Could you check a few things on this model? Use its own coordinates, in mm. A direction names the side the tool comes from. Give positions to 0.01 mm unless a question says otherwise; leave off trailing zeros. Order: outer loops, then holes, each group sorted by start corner. A loop starts at its lowest first (then second) coordinate and runs counter-clockwise, first axis right, second up. Notation, with made-up numbers: (37.5, 11.5) -> (85.5, 11.5) arc R19 ccw to (85.5, 39.5) -> close; hole circle Ø5 at (-23, -12). An arc over 180 degrees is marked (long way). Use one line per item in the form item = value. Start each with the question number.
from build123d import *

# Parameters (mm, degrees)
SKETCH1_R           = 76.2
BOSS_EXTRUDE1_DEPTH = 16.256
SHELL1_T            = -3.175
FILLET1_R           = 1.5875
SKETCH2_R           = 38.1
CUT_EXTRUDE1_DEPTH  = 16.256
SKETCH3_R           = 1.524
CUT_EXTRUDE2_DEPTH  = 76.2
CIRPATTERN1_COUNT   = 6
CUT_EXTRUDE4_START  = -1.524
SKETCH5_R           = 76.2
CUT_EXTRUDE4_DEPTH  = 1.524


with BuildPart() as part:
    # Sketch1 → Boss-Extrude1 (new body)
    with BuildSketch(Plane(origin=(0, 0, 0), x_dir=(1, 0, 0), z_dir=(0, 1, 0))):
        with Locations(Location((0, 0, 0), (0, 0, 270))):
            Circle(SKETCH1_R)
    extrude(amount=BOSS_EXTRUDE1_DEPTH)

    # Shell1
    shell1_openings = [part.faces().sort_by_distance(p)[0] for p in [
        (0, 16.256, 0),
    ]]
    offset(amount=SHELL1_T, openings=shell1_openings, kind=Kind.INTERSECTION)

    # Fillet1
    fillet1_edges = [part.edges().sort_by_distance(p)[0] for p in [
        (0, 3.175, -73.025),
    ]]
    fillet(fillet1_edges, radius=FILLET1_R)

    # Sketch2 → Cut-Extrude1 (cut)
    with BuildSketch(Plane.XZ):
        with Locations(Location((0, 0, 0), (0, 0, 270))):
            Circle(SKETCH2_R)
    extrude(amount=-CUT_EXTRUDE1_DEPTH, mode=Mode.SUBTRACT)

    # Sketch3 → Cut-Extrude2 (cut)
    with BuildSketch(Plane(origin=(0, 0, 0), x_dir=(0, 0, -1), z_dir=(1, 0, 0))):
        with Locations((0, 8.636)):
            Circle(SKETCH3_R)
    cut_extrude2 = extrude(amount=-CUT_EXTRUDE2_DEPTH, mode=Mode.SUBTRACT)

    # CirPattern1: Cut-Extrude2 ×6 about axis
    cirpattern1_axis = Axis((0, 16.256, 0), (0, -1, 0))
    for i in range(1, CIRPATTERN1_COUNT):
        add(cut_extrude2.rotate(cirpattern1_axis, i * 360 / CIRPATTERN1_COUNT), mode=Mode.SUBTRACT)

    # Sketch5 → Cut-Extrude4 (cut)
    with BuildSketch(Plane(origin=(0, 16.256, 0), x_dir=(1, 0, 0), z_dir=(0, 1, 0)).offset(CUT_EXTRUDE4_START)):
        with Locations(Location((0, 0, 0), (0, 0, 270))):
            Circle(SKETCH5_R)
    extrude(amount=CUT_EXTRUDE4_DEPTH, mode=Mode.SUBTRACT)


solid = part.part
(1) Imagine slicing it at A-A (x = 0). Write out the boundary of the cut face in (y, z) (1 decimal).
(2) Please list where these lines run through material, in increasing order: probe 1 along Y at (x, z) = (-73.95, 0); probe 2 along X at (y, z) = (14.25, -1); probe 3 along Y at (x, z) = (31.5, 46) (3 decimals).
(3) I'm going to push flat-ended pins straight in: pin 1 Ø5 at (x, y) = (42, 1.5) entering from -Z; pin 2 Ø3 at (x, z) = (55.5, -30.5) entering from -Y; pin 3 Ø4 at (y, z) = (6, 59.5) entering from +X; pin 4 Ø5 at (x, y) = (-58.5, 9.5) entering from -Z. Where does each tip first touch, or does it pass through?
(4) We'd pull the mould along Y, two halves only. Please class faces 1 (the cylindrical face through (38.61, 8.7, 63.83)), 2 (the cylindrical face through (37.9, 7.284, -64.238)), 3 (the cylindrical face through (-23.183, 1.565, 30.235)), 4 (the flat face through (-16, 0, -35)): pulls with the +Y half, pulls with the -Y half, needs draft (parallel to the pull), parting line crosses it, or undercut.
(5) Imagine slicing it at B-B (y = 13). Write out the boundary of the cut face in (x, z) (3 decimals).
(6) Which directions (+Z, -Z, +X, -X, +Y, -Y) give clear straight access to the entire face, cutting with the end or side of a thin tool? Please do faces 5 (the cylindrical face through (-37.9, 7.284, 64.238)), 6 (the cylindrical face through (21.935, 9.677, 69.653)).
Calculated:
q1.outline = (0, -76.2) -> (14.7, -76.2) -> (14.7, -73) -> (4.8, -73) arc R1.6 cw to (3.2, -71.4) -> (3.2, -38.1) -> (0, -38.1) -> close; (0, 38.1) -> (3.2, 38.1) -> (3.2, 71.4) arc R1.6 cw to (4.8, 73) -> (14.7, 73) -> (14.7, 76.2) -> (0, 76.2) -> close
q2.probe_1 = 0 to 7.11, 10.16 to 14.73
q2.probe_2 = -76.19 to -73.02, 73.02 to 76.19
q2.probe_3 = 0 to 3.175
q3.pin_1 = -65.16
q3.pin_2 = 0
q3.pin_3 = 50
q3.pin_4 = -51.68
q4.face_1 = undercut
q4.face_2 = undercut
q4.face_3 = needs draft
q4.face_4 = pulls with the -Y half
q5.outline = circle Ø152.4 at (0, 0); hole circle Ø146.05 at (0, 0)
q6.face_5 = none
q6.face_6 = +Y
